Source: CAD feature listing. Evaluate the final solid. Frame: model axes, mm. Give positions to 0.01 mm unless a question says otherwise; leave off trailing zeros. Write each loop counter-clockwise with the first axis right and the second up, starting at its lowest first coordinate (ties: lowest second). Pieces come first, ordered by that corner, then holes. Notation, with made-up numbers: (-16.5, 56) -> (14.5, 56) arc R25 cw to (14.5, 73) -> close; hole circle Ø10 at (3.25, 65.5). An arc over 180 degrees is marked (long way). Answer as a JSON object with one key per item and string values. Group by question number.
Item 1: Ray query, probe 1 along X at (y, z) = (-10.5, 4.65); probe 2 along Y at (x, z) = (90, 2.3); probe 3 along X at (y, z) = (-12, 0.8). Return the intervals inside material, ascending. Write a range as from..to.
Item 2: Section query A-A on z = 2.7. Return the cut outline in (x, y).
Item 3: Pull-direction query (Y, two-part tool) for faces 1 (the face through (-2, 0, 0)), 2 (the face through (-134.76, -13.95, 2.46)), 3 (the face through (-2, 27, 2)); classes: pulls with the +Y half, pulls with the -Y half, needs draft (parallel to the pull), parting line crosses it, or undercut.
Item 4: Section query B-B on x = 90. Return the cut outline in (y, z).
from build123d import *

# Parameters (mm, degrees)
SKETCH_1_W          = 300
SKETCH_1_H          = 54
EXTRUDE_1_DEPTH     = 5
SKETCH_2_R          = 6
CUT_EXTRUDE_1_DEPTH = 6
SKETCH_3_R          = 6.5
CUT_EXTRUDE_2_DEPTH = 10


with BuildPart() as part:
    # 草图1 → 凸台-拉伸1 (new body)
    with BuildSketch(Plane.XY):
        Rectangle(SKETCH_1_W, SKETCH_1_H)
    extrude(amount=EXTRUDE_1_DEPTH)

    # 草图2 → 切除-拉伸1 (cut, through all)
    with BuildSketch(Plane(origin=(0, 0, 0), x_dir=(-1, 0, 0), z_dir=(0, 0, -1))):
        with Locations((-130, -10.3)):
            Circle(SKETCH_2_R)
    cut_extrude_1 = extrude(amount=-CUT_EXTRUDE_1_DEPTH, mode=Mode.SUBTRACT)

    # 镜向1: 切除-拉伸1 across plane
    add(cut_extrude_1.mirror(Plane(origin=(0, 0, 0), x_dir=(0, 0, 1), z_dir=(1, 0, 0))), mode=Mode.SUBTRACT)

    # 草图3 → 切除-拉伸2 (cut)
    with BuildSketch(Plane(origin=(0, 0, 0), x_dir=(-1, 0, 0), z_dir=(0, 0, -1))):
        with Locations((-90, -10)):
            Circle(SKETCH_3_R)
    cut_extrude_2 = extrude(amount=-CUT_EXTRUDE_2_DEPTH, mode=Mode.SUBTRACT)

    # 镜向2: 切除-拉伸2 across plane
    add(cut_extrude_2.mirror(Plane(origin=(0, 0, 0), x_dir=(0, 0, 1), z_dir=(1, 0, 0))), mode=Mode.SUBTRACT)


solid = part.part
Worked answers:
{
 "1": {"probe 1": "-150..-136, -124..-96.48, -83.52..83.52, 96.48..124, 136..150", "probe 2": "-27..-16.5, -3.5..27", "probe 3": "-150..-135.75, -124.25..-96.18, -83.82..83.82, 96.18..124.25, 135.75..150"},
 "2": {"outline": "(-150, -27) -> (150, -27) -> (150, 27) -> (-150, 27) -> close; hole circle Ø12 at (-130, -10.3); hole circle Ø13 at (-90, -10); hole circle Ø13 at (90, -10); hole circle Ø12 at (130, -10.3)"},
 "3": {"face 1": "needs draft", "face 2": "undercut", "face 3": "pulls with the +Y half"},
 "4": {"outline": "(-27, 0) -> (-16.5, 0) -> (-16.5, 5) -> (-27, 5) -> close; (-3.5, 0) -> (27, 0) -> (27, 5) -> (-3.5, 5) -> close"}
}
